For this review, take the finished solid that the model builds, in its own axes (mm). A direction names the side the tool comes from. Coordinates: 2 decimals unless noted, no trailing zeros. Loops run counter-clockwise (first coordinate to the right, second up) from the corner with the lowest first, then second, coordinate; pieces in that order, holes last. Notation, with made-up numbers: M 69,1.25 L 116,1.25 A17 ccw 116,24.25 Z; hole C -1,-24.75 d6. An arc over 180 degrees is marked long. Use one line per item in the form item = value.
Autodesk Inventor part; units mm, degrees
ref_plane "YZ Plane" through (0, 0, 0) normal (1, 0, 0) x (0, 1, 0)
ref_plane "XZ Plane" through (0, 0, 0) normal (0, 1, 0) x (-1, 0, 0)
ref_plane "XY Plane" through (0, 0, 0) normal (0, 0, 1) x (1, 0, 0)
sketch "Sketch1" plane through (0, 0, 0) normal (1, 0, 0) x (0, 1, 0)
  line L0 (0, 0) -> (76.2, 0)
  line L1 (76.2, 0) -> (76.2, -76.2)
  line L2 (76.2, -76.2) -> (0, -76.2)
  line L3 (0, -76.2) -> (0, 0)
  line L4 (20.4851, -17.6149) -> (55.7149, -17.6149)
  line L5 (55.7149, -17.6149) -> (55.7149, -55.7149)
  line L6 (55.7149, -55.7149) -> (20.4851, -55.7149)
  line L7 (20.4851, -55.7149) -> (20.4851, -17.6149)
  line L8 (20.4851, -17.6149) -> (55.7149, -55.7149) construction
  line L9 (55.7149, -17.6149) -> (20.4851, -55.7149) construction
  line L10 (76.2, 0) -> (55.7149, -17.6149)
  line L11 (20.4851, -55.7149) -> (0, -76.2)
  line L12 (0, 0) -> (20.4851, -17.6149)
  line L13 (55.7149, -55.7149) -> (76.2, -76.2)
  circle A0 centre (65.9575, -8.8074) radius 2.5
  circle A1 centre (65.9575, -65.9574) radius 2.5
  circle A2 centre (10.2426, -65.9575) radius 2.5
  circle A3 centre (10.2426, -8.8074) radius 2.5
  line L14 (29.5453, -27.4133) -> (46.6547, -27.4133)
  line L15 (46.6547, -27.4133) -> (46.6547, -45.9165)
  line L16 (46.6547, -45.9165) -> (29.5453, -45.9165)
  line L17 (29.5453, -45.9165) -> (29.5453, -27.4133)
  line L18 (29.5453, -27.4133) -> (46.6547, -45.9165) construction
  line L19 (46.6547, -27.4133) -> (29.5453, -45.9165) construction
  point P0 (38.1, -36.6649)
  dimension "d0" = 76.2
  dimension "d1" = 76.2
  dimension "d2" = 35.2298
  dimension "d3" = 38.1
  dimension "d4" = 5
  dimension "d5" = 5
  dimension "d6" = 5
  dimension "d7" = 5
  dimension "d8" = 49.308
  dimension "d9" = 29.5453
extrude "Extrusion1" add sketch "Sketch1" along normal blind 5
extrude "Extrusion2" cut sketch "Sketch1" along normal blind 5 contours A3 L12 | L12 A3 | A0 L10 | L10 A0 | A2 L11 | L11 A2 | A1 L13 | L13 A1
sketch "Sketch2" plane through (5, 0, 0) normal (1, 0, 0) x (0, 0, -1)
  line L0 (76.2, 0) -> (76.2, 76.2)
  line L1 (27.4133, 29.5453) -> (76.2, 0)
  line L2 (45.9165, 29.5453) -> (0, 0)
  circle A0 centre (36.9453, 23.7727) radius 2.5
  line L3 (36.9453, 23.7727) -> (36.9453, 0)
  dimension "d14" = 5
  dimension "d19" = 23.7727
extrude "Extrusion3" cut sketch "Sketch2" against normal blind 25.4
thread "Thread1"
properties part number "plateform du bas"
1. For pin 1 Ø4 at (y, z) = (23.77, -36.95) entering from -X, flat-tipped, find the tip position at first contact; note if it passes through.
Computed values:
pin_1 = through
2. Consider section A-A on y = 32. Write out the cut boundary in (x, z).
Computed values:
outline = M 0,-76.2 L 5,-76.2 L 5,-45.92 L 0,-45.92 Z; M 0,-27.41 L 5,-27.41 L 5,0 L 0,0 Z
3. Consider section D-D on z = -7.5. Write out the cut boundary in (x, y), plus the area to 3 significant figures.
Computed values:
outline = M 0,0 L 5,0 L 5,8.11 L 0,8.11 Z; M 0,12.37 L 5,12.37 L 5,63.83 L 0,63.83 Z; M 0,68.09 L 5,68.09 L 5,76.2 L 0,76.2 Z
area = 338 mm2
4. Tool access review of faces 5 (the face through (2, 38, -45.916)), 6 (the face through (2, 0, -39)): name each direction out of +Z, -Z, +X, -X, +Y, -Y from which nothing blocks a thin tool from reaching the whole face with its end or side.
Computed values:
face_5 = +X, -X
face_6 = +Z, -Z, +X, -X, -Y
5. Consider section B-B on z = -32. Write out the cut boundary in (x, y).
Computed values:
outline = M 0,0 L 5,0 L 5,29.55 L 0,29.55 Z; M 0,46.65 L 5,46.65 L 5,76.2 L 0,76.2 Z
6. Wall thickness on line 1 along Y through (x, z) = (2.8, -27.5); line 2 along Y through (x, z) = (2.75, -37.5); line 3 along Z through (x, y) = (1.1, 64): over which ranges is each line inside the solid? List them lowest first. Write a range as from..to.
Computed values:
line_1 = 0..29.55, 46.65..76.2
line_2 = 0..21.34, 26.21..29.55, 46.65..76.2
line_3 = -76.2..-67.51, -64.4..-10.36, -7.25..0
7. Consider section C-C on x = 4.15. Write out the cut boundary in (y, z).
Computed values:
outline = M 0,-76.2 L 76.2,-76.2 L 76.2,0 L 0,0 Z; hole C 10.24,-65.96 d5; hole C 10.24,-8.81 d5; hole C 23.77,-36.95 d5; hole M 29.55,-45.92 L 46.65,-45.92 L 46.65,-27.41 L 29.55,-27.41 Z; hole C 65.96,-65.96 d5; hole C 65.96,-8.81 d5
8. Draft analysis for pull direction Z (two halves, no side actions). For faces 1 (the face through (0, 29, -38)), 2 (the face through (2, 39, -76.2)), 3 (the face through (2.465, 12.627, -9.558)), 4 (the face through (2, 38, -27.413)), state which applies: +Z half, -Z half, draft (parallel to the pull), parting line (faces both ways), or undercut.
Computed values:
face_1 = draft
face_2 = -Z half
face_3 = undercut
face_4 = undercut
